Here's the drawing with two shaded views (mm, measured from the low corner). I have some questions. A direction names the side the tool comes from. Give positions to 0.01 mm unless a question says otherwise; leave off trailing zeros. Write each loop counter-clockwise with the first axis right and the second up, starting at its lowest first coordinate (ties: lowest second). Pieces come first, ordered by that corner, then holes. Notation, with made-up numbers: (18.25, 28) -> (41.25, 28) arc R21 ccw to (41.25, 58) -> close; hole circle Ø8 at (-15.5, -39). An arc over 180 degrees is marked (long way). One line per question, with ' | ' between items.
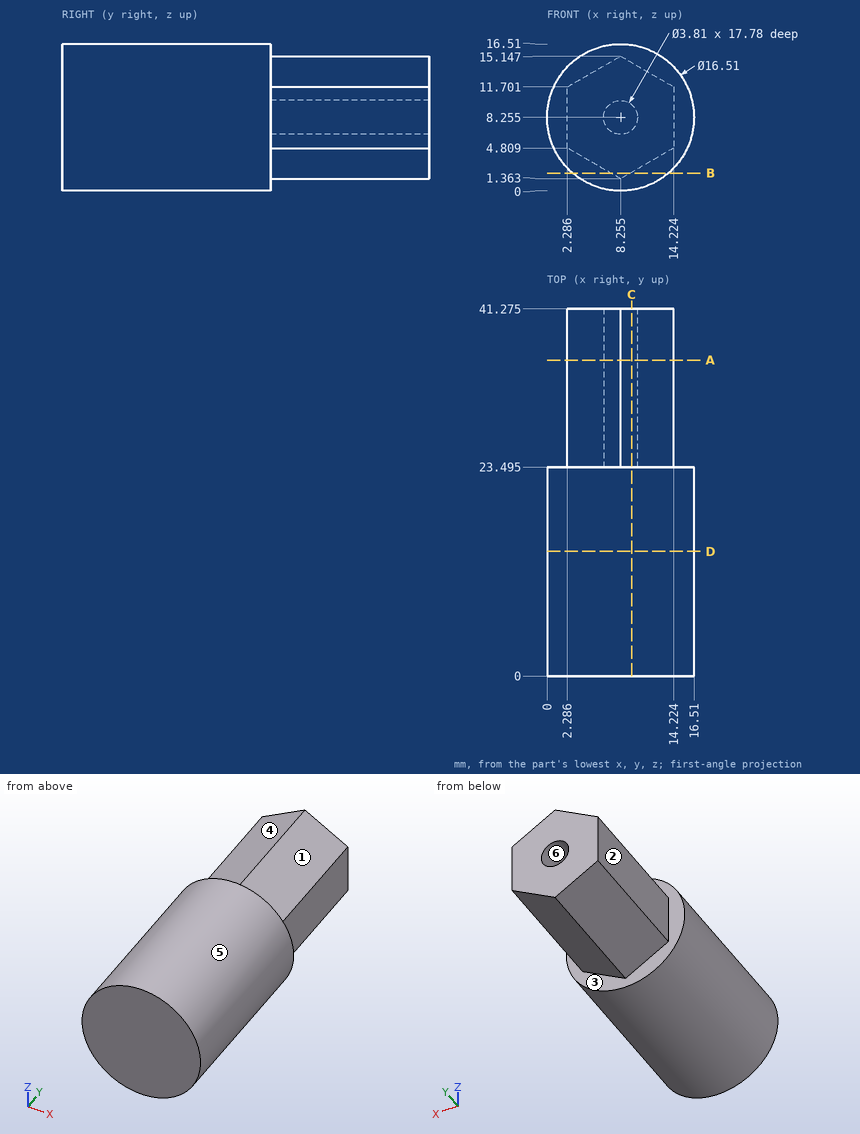
Q1. Imagine slicing it at B-B on z = 2. Please give me the cut outline in (x, y) (1 decimal).
Answer below:
outline: (2.9, 0) -> (13.6, 0) -> (13.6, 23.5) -> (9.4, 23.5) -> (9.4, 41.3) -> (7.2, 41.3) -> (7.2, 23.5) -> (2.9, 23.5) -> close
Q2. On a 3-axis mill with a long thin cutter (end or side, diameter ignored), from which of +Z, -Z, +X, -X, +Y, -Y can I reach the whole of each face in a straight line? I mean the marked faces 1, 2 and 3. Say none if no direction works.
Answer below:
face 1: +Z, +X, +Y | face 2: +Z, -Z, -X, +Y | face 3: +Y
Q3. Imagine slicing it at A-A on y = 35.5. Please give me the cut outline in (x, z) (1 decimal), and give its area (3 significant figures).
Answer below:
outline: (2.3, 4.8) -> (8.3, 1.4) -> (14.2, 4.8) -> (14.2, 11.7) -> (8.3, 15.1) -> (2.3, 11.7) -> close; hole circle Ø3.8 at (8.3, 8.3) | area: 112 mm^2
Q4. Imagine slicing it at C-C on x = 9.5. Please give me the cut outline in (y, z) (1 decimal), and give its area (3 significant figures).
Answer below:
outline: (0, 0.1) -> (23.5, 0.1) -> (23.5, 2.1) -> (41.3, 2.1) -> (41.3, 6.8) -> (23.5, 6.8) -> (23.5, 9.7) -> (41.3, 9.7) -> (41.3, 14.4) -> (23.5, 14.4) -> (23.5, 16.4) -> (0, 16.4) -> close | area: 552 mm^2
Q5. If we mould it in two halves opening along Z, with no side actions, what happens to the marked faces 4, 5 and 6? For each: +Z half, -Z half, draft (parallel to the pull), parting line (faces both ways), or undercut.
Answer below:
face 4: +Z half | face 5: parting line | face 6: undercut
Q6. Will these pins go through, and if not, where does the flat tip stop? pin 1 (1.5 mm diameter, centred on x = 14.5, y = 25, fed in from +Z) (1 decimal); pin 2 (7.5 mm diameter, centred on y = 29.5, z = 7.5, fed in from +X); pin 3 (1.1 mm diameter, centred on x = 7.5, z = 8, fed in from +Y) (3 decimals).
Answer below:
pin 1: stops at z = 12 | pin 2: stops at x = 14.22 | pin 3: stops at y = 23.495
Q7. If I drill on line 1 along Z through (x, y) = (8, 18); line 2 along Y through (x, z) = (7, 0.5) (1 decimal); line 3 along X through (y, z) = (32, 8.5) (1 decimal), over which ranges is the centre line in solid material (lowest first)?
Answer below:
line 1: z = 0 to 16.51 | line 2: y = 0 to 23.5 | line 3: x = 2.3 to 6.4, 10.1 to 14.2
Q8. Imagine slicing it at D-D on y = 14. Please give me the cut outline in (x, z) (1 decimal).
Answer below:
outline: circle Ø16.5 at (8.3, 8.3)
